The listing builds one solid part. Answer for the finished solid, in the listing's coordinates (mm). A direction names the side the tool comes from. Round coordinates to 2 decimals unless told otherwise and drop trailing zeros. Write each loop counter-clockwise with the first axis right and the second up, starting at its lowest first coordinate (ties: lowest second). Pieces come first, ordered by that corner, then holes.
(1) A cutting plane is placed at D-D, the plane y = 53. Give the vertices of the cut face in (x, z), and give its area (3 significant figures).
(2) A cutting plane is placed at B-B, the plane y = 3.5. Give the vertices of the cut face in (x, z).
(3) A cutting plane is placed at A-A, the plane x = 0.5. Give the vertices of the cut face in (y, z).
(4) A cutting plane is placed at C-C, the plane z = 1.5. Give the vertices of the cut face in (x, y), and give its area (3 significant figures).
(5) For faces 1 (the face through (0, -14, -4)), 2 (the face through (0, 10, -3)), 3 (the face through (3.25, 5, -3)), 4 (the face through (-2.75, -14, -5)), determine the directions among +Z, -Z, +X, -X, +Y, -Y from which every point of the face is accessible in a straight line to the end or side of a thin tool.
(6) Each of these flat-tipped pins is pushed along its axis until it touches: pin 1 Ø6 at (x, y) = (1, 31) entering from -Z; pin 2 Ø0.6 at (y, z) = (-11.5, -5) entering from +X; pin 3 Ø4 at (x, z) = (-2.5, 3) entering from -Y; pin 4 Ø5.5 at (x, z) = (2.5, -2.5) entering from -Y. Where does it stop, or does it pass through?
(7) Find the intervals of material crossed by probe 1 along Z at (x, y) = (-0.25, 13.5); probe 2 along Z at (x, y) = (0.75, -17); probe 3 along Y at (x, z) = (0, -5.5), in increasing order.
from build123d import *

# Parameters (mm, degrees)
SKETCH_W     = 13.34
SKETCH_H     = 90
PAD_DEPTH    = 5
SKETCH001_W  = 6.5
SKETCH001_H  = 10
PAD001_DEPTH = 6
SKETCH002_W  = 5.5
SKETCH002_H  = 2
PAD002_DEPTH = 29


with BuildPart() as part:
    # Sketch → Pad (new body)
    with BuildSketch(Plane.XY):
        with Locations((0, 45)):
            Rectangle(SKETCH_W, SKETCH_H)
    extrude(amount=PAD_DEPTH)

    # Sketch001 (on Face5 of Pad) → Pad001 (join)
    with BuildSketch(Plane(origin=(0, 0, 0), x_dir=(1, 0, 0), z_dir=(0, 0, -1))):
        with Locations((0, -5)):
            Rectangle(SKETCH001_W, SKETCH001_H)
    extrude(amount=PAD001_DEPTH)

    # Sketch002 (on Face5 of Pad001) → Pad002 (join)
    with BuildSketch(Plane.XZ):
        with Locations((0, -5)):
            Rectangle(SKETCH002_W, SKETCH002_H)
    extrude(amount=PAD002_DEPTH)


solid = part.part
Solutions:
1. outline: (-6.67, 0) - (6.67, 0) - (6.67, 5) - (-6.67, 5) - close
1. area: 66.7 mm2
2. outline: (-6.67, 0) - (-3.25, 0) - (-3.25, -6) - (3.25, -6) - (3.25, 0) - (6.67, 0) - (6.67, 5) - (-6.67, 5) - close
3. outline: (-29, -6) - (10, -6) - (10, 0) - (90, 0) - (90, 5) - (0, 5) - (0, -4) - (-29, -4) - close
4. outline: (-6.67, 0) - (6.67, 0) - (6.67, 90) - (-6.67, 90) - close
4. area: 1,200 mm2
5. face 1: +Z, +X, -X, -Y
5. face 2: -Z, +X, -X, +Y
5. face 3: -Z, +X, +Y, -Y
5. face 4: +Z, -Z, -X, -Y
6. pin 1: stops at z = 0
6. pin 2: stops at x = 2.75
6. pin 3: stops at y = 0
6. pin 4: stops at y = -29
7. probe 1: z = 0 to 5
7. probe 2: z = -6 to -4
7. probe 3: y = -29 to 10
